Read the model definition and answer for the solid it produces. Units are mm, in the model's axes. Give positions to 0.01 mm unless a question says otherwise; leave off trailing zeros. Order: outer loops, then holes, each group sorted by start corner. A loop starts at its lowest first (then second) coordinate and runs counter-clockwise, first axis right, second up. Notation, with made-up numbers: (7.25, 51.5) - (26.25, 51.5) arc R15 cw to (26.25, 67.5) - close; hole circle Ø8 at (64.25, 55). An arc over 180 degrees is marked (long way). Write each question's results on one line, items separated by ' | '.
from build123d import *

# Parameters (mm, degrees)
F0_W     = 161.985158
F0_H     = 94.046846
F0_R     = 42.376618
F1_DEPTH = 15.494
F2_R     = 2.54


with BuildPart() as f1:
    # F0 (on Top) → F1 (new body)
    with BuildSketch(Plane.XY):
        Rectangle(F0_W, F0_H)
        with Locations((-2.667, 0)):
            Circle(F0_R, mode=Mode.SUBTRACT)
    extrude(amount=F1_DEPTH)

    # F2
    f2_edges = [f1.edges().sort_by_distance(p)[0] for p in [
        (-45.043619, 0, 15.494),
    ]]
    fillet(f2_edges, radius=F2_R)


solid = f1.part
(1) The mould has two halves that part along Y. Classify faces 1 (the face through (17, 42, 15.494)), 2 (the face through (-1, 47.023, 8)), 3 (the face through (-36.296, -25.786, 6.386)): pulls with the +Y half, pulls with the -Y half, needs draft (parallel to the pull), parting line crosses it, or undercut.
Conclusion:
face 1: needs draft | face 2: pulls with the +Y half | face 3: undercut
(2) Section B-B (z = 3) is taken. Give the vertices of the cut face in (x, y), plus the area to 3 significant figures.
Conclusion:
outline: (-80.99, -47.02) - (80.99, -47.02) - (80.99, 47.02) - (-80.99, 47.02) - close; hole circle Ø84.75 at (-2.67, 0) | area: 9,590 mm^2
(3) Section A-A (y = 0) is taken. Give the vertices of the cut face in (x, z), plus the area to 3 significant figures.
Conclusion:
outline: (-80.99, 0) - (-45.04, 0) - (-45.04, 12.95) arc R2.54 ccw to (-47.58, 15.49) - (-80.99, 15.49) - close; (39.71, 0) - (80.99, 0) - (80.99, 15.49) - (42.25, 15.49) arc R2.54 ccw to (39.71, 12.95) - close | area: 1,190 mm^2
(4) Consider probe 1 along Y at (x, z) = (-20, 7); probe 2 along Y at (x, z) = (22, 9); probe 3 along X at (y, z) = (37.5, 10.5). Determine where each line is inside the solid, lowest interval first. Write a range as [from, to].
Conclusion:
probe 1: [-47.02, -38.67], [38.67, 47.02] | probe 2: [-47.02, -34.46], [34.46, 47.02] | probe 3: [-80.99, -22.4], [17.07, 80.99]
